Work out the finished part from the listing and answer in its coordinate system (mm). A direction names the side the tool comes from. Coordinates: 2 decimals unless noted, no trailing zeros. Loops run counter-clockwise (first coordinate to the right, second up) from the corner with the lowest first, then second, coordinate; pieces in that order, holes last. Notation, with made-up numbers: M 78,-13.5 L 136,-13.5 A24 ccw 136,20.5 Z; hole C 59.5,26.25 d8. An arc over 180 degrees is marked long. Write each question's results on one line, items separated by ' | '.
```python
from build123d import *

# Parameters (mm, degrees)
EXTRUDE1_DEPTH             = 75.692
SKETCH2_W                  = 7.9502
SKETCH2_H                  = 18.2626
SKETCH2_W_2                = 7.9248
EXTRUDE2_DEPTH             = 33.4772
EXTRUDE3_REACH             = 33.89
SKETCH3_W                  = 59.817
SKETCH3_H                  = 1.5875
EXTRUDE3_DIRECTION_2_REACH = 3.588
SKETCH4_W                  = 3.175
SKETCH4_H                  = 6.3373
EXTRUDE4_DEPTH             = 1.5875
SKETCH5_R                  = 4.0005
SKETCH5_R_2                = 1.1938
SKETCH5_R_3                = 2.1844
EXTRUDE5_DEPTH             = 1.5875
SKETCH6_R                  = 2.1844
SKETCH6_R_2                = 1.5875
EXTRUDE6_DEPTH             = 43.8498
FILLET1_R                  = 2.54
FILLET2_R                  = 0.254
FILLET3_R                  = 2.54
FILLET4_R                  = 2.54


with BuildPart() as part:
    # Sketch1 → Extrude1 (new body)
    with BuildSketch(Plane(origin=(0, 0, 0), x_dir=(0, 0, -1), z_dir=(1, 0, 0))):
        with BuildLine():
            Line((1.5875, 33.4772), (1.5875, 1.5875))
            Line((1.5875, 1.5875), (41.2623, 1.5875))
            Line((41.2623, 1.5875), (41.2623, 33.4772))
            Line((41.2623, 33.4772), (42.8498, 33.4772))
            Line((42.8498, 33.4772), (42.8498, 1.5875))
            ThreePointArc((42.8498, 1.5875), (42.384832015, 0.464967985), (41.2623, 0))
            Line((41.2623, 0), (1.5875, 0))
            ThreePointArc((1.5875, 0), (0.464967985, 0.464967985), (0, 1.5875))
            Line((0, 1.5875), (0, 33.4772))
            Line((0, 33.4772), (1.5875, 33.4772))
        make_face()
    extrude(amount=EXTRUDE1_DEPTH)

    # Sketch2 → Extrude2 (cut)
    with BuildSketch(Plane(origin=(0, 33.4772, 0), x_dir=(1, 0, 0), z_dir=(0, 1, 0))):
        with Locations((3.9751, 9.1313)):
            Rectangle(SKETCH2_W, SKETCH2_H)
        with Locations((71.7296, 9.1313)):
            Rectangle(SKETCH2_W_2, SKETCH2_H)
    extrude(amount=-EXTRUDE2_DEPTH, mode=Mode.SUBTRACT)

    # Extrude3: up to this face of the body (flat: up to its plane)
    extrude3_end = Plane(part.part.faces().sort_by_distance((37.846, 33.4772, -42.05605))[0])
    # Sketch3 → Extrude3 (cut, up to the picked face)
    with BuildSketch(Plane(origin=(0, 1.5875, 0), x_dir=(1, 0, 0), z_dir=(0, 1, 0)), mode=Mode.PRIVATE) as extrude3_sk1:
        with Locations((37.8587, 42.05605)):
            Rectangle(SKETCH3_W, SKETCH3_H)
    extrude3_tool1 = split(extrude(extrude3_sk1.sketch, amount=EXTRUDE3_REACH, mode=Mode.PRIVATE), bisect_by=extrude3_end, keep=Keep.BOTH, mode=Mode.PRIVATE)
    add(extrude3_tool1.solids().sort_by(Axis((37.8587, 1.5875, -42.05605), (0, 1, 0)))[0], mode=Mode.SUBTRACT)

    # Extrude3 direction 2: up to this face of the body (flat: up to its plane)
    extrude3_direction_2_end = Plane(part.part.faces().sort_by_distance((37.850626027, 0, -22.536595268))[0])
    # Sketch3 → Extrude3 direction 2 (cut, up to the picked face)
    with BuildSketch(Plane(origin=(0, 1.5875, 0), x_dir=(1, 0, 0), z_dir=(0, 1, 0)), mode=Mode.PRIVATE) as extrude3_direction_2_sk1:
        with Locations((37.8587, 42.05605)):
            Rectangle(SKETCH3_W, SKETCH3_H)
    extrude3_direction_2_tool1 = split(extrude(extrude3_direction_2_sk1.sketch, amount=-EXTRUDE3_DIRECTION_2_REACH, mode=Mode.PRIVATE), bisect_by=extrude3_direction_2_end, keep=Keep.BOTH, mode=Mode.PRIVATE)
    add(extrude3_direction_2_tool1.solids().sort_by(Axis((37.8587, 1.5875, -42.05605), (0, -1, 0)))[0], mode=Mode.SUBTRACT)

    # Sketch4 → Extrude4 (cut)
    with BuildSketch(Plane(origin=(0, 1.5875, 0), x_dir=(1, 0, 0), z_dir=(0, 1, 0))):
        with Locations((9.5377, 38.09365)):
            Rectangle(SKETCH4_W, SKETCH4_H)
        with Locations((66.1797, 38.09365)):
            Rectangle(SKETCH4_W, SKETCH4_H)
    extrude(amount=-EXTRUDE4_DEPTH, mode=Mode.SUBTRACT)

    # Sketch5 → Extrude5 (cut)
    with BuildSketch(Plane(origin=(0, 1.5875, 0), x_dir=(1, 0, 0), z_dir=(0, 1, 0))):
        with Locations(Location((21.1836, 29.1592, 0), (0, 0, 270))):  # turned: the seam where the file's is
            Circle(SKETCH5_R)
        with Locations(Location((21.1836, 37.4904, 0), (0, 0, 270))):  # turned: the seam where the file's is
            Circle(SKETCH5_R_2)
        with Locations(Location((12.8524, 29.1592, 0), (0, 0, 270))):  # turned: the seam where the file's is
            Circle(SKETCH5_R_2)
        with Locations(Location((21.1836, 20.828, 0), (0, 0, 270))):  # turned: the seam where the file's is
            Circle(SKETCH5_R_2)
        with Locations(Location((37.846, 37.4904, 0), (0, 0, 270))):  # turned: the seam where the file's is
            Circle(SKETCH5_R_2)
        with Locations(Location((29.5148, 29.1592, 0), (0, 0, 270))):  # turned: the seam where the file's is
            Circle(SKETCH5_R_2)
        with Locations(Location((37.846, 20.828, 0), (0, 0, 270))):  # turned: the seam where the file's is
            Circle(SKETCH5_R_2)
        with Locations(Location((37.846, 29.1592, 0), (0, 0, 270))):  # turned: the seam where the file's is
            Circle(SKETCH5_R)
        with Locations(Location((54.5084, 20.828, 0), (0, 0, 270))):  # turned: the seam where the file's is
            Circle(SKETCH5_R_2)
        with Locations(Location((54.5084, 29.1592, 0), (0, 0, 270))):  # turned: the seam where the file's is
            Circle(SKETCH5_R)
        with Locations(Location((46.1772, 29.1592, 0), (0, 0, 270))):  # turned: the seam where the file's is
            Circle(SKETCH5_R_2)
        with Locations(Location((54.5084, 37.4904, 0), (0, 0, 270))):  # turned: the seam where the file's is
            Circle(SKETCH5_R_2)
        with Locations(Location((62.8396, 29.1592, 0), (0, 0, 270))):  # turned: the seam where the file's is
            Circle(SKETCH5_R_2)
        with Locations(Location((3.7592, 29.1592, 0), (0, 0, 270))):  # turned: the seam where the file's is
            Circle(SKETCH5_R_3)
        with Locations(Location((71.9328, 29.1592, 0), (0, 0, 270))):  # turned: the seam where the file's is
            Circle(SKETCH5_R_3)
    extrude(amount=-EXTRUDE5_DEPTH, mode=Mode.SUBTRACT)

    # Sketch6 → Extrude6 (cut, through all)
    with BuildSketch(Plane.XY):
        with Locations((3.7592, 27.0002)):
            Circle(SKETCH6_R)
        with Locations((3.7592, 11.1252)):
            Circle(SKETCH6_R)
        with Locations((71.9328, 27.0002)):
            Circle(SKETCH6_R)
        with Locations((71.9328, 11.1252)):
            Circle(SKETCH6_R)
        with Locations((22.0726, 19.05)):
            Circle(SKETCH6_R_2)
        with Locations((53.6194, 19.05)):
            Circle(SKETCH6_R_2)
    extrude(amount=-EXTRUDE6_DEPTH, mode=Mode.SUBTRACT)

    # Fillet1
    fillet1_edges = [part.edges().sort_by_distance(p)[0] for p in [
        (64.5922, 0.79375, -41.2623),
        (0, 33.4772, -42.05605),
        (7.9502, 33.4772, -0.79375),
        (75.692, 33.4772, -42.05605),
        (75.692, 0.79375, -18.2626),
        (67.7672, 33.4772, -0.79375),
        (11.1252, 0.79375, -41.2623),
    ]]
    fillet(fillet1_edges, radius=FILLET1_R)

    # Fillet2
    fillet2_edges = [part.edges().sort_by_distance(p)[0] for p in [
        (71.7296, 1.5875, -41.2623),
        (37.8587, 1.5875, -1.5875),
        (3.9751, 1.5875, -41.2623),
    ]]
    fillet(fillet2_edges, radius=FILLET2_R)

    # Fillet3
    fillet3_edges = [part.edges().sort_by_distance(p)[0] for p in [
        (0, 0.79375, -18.2626),
    ]]
    fillet(fillet3_edges, radius=FILLET3_R)

    # Fillet4
    fillet4_edges = [part.edges().sort_by_distance(p)[0] for p in [
        (67.7672, 33.4772, -42.05605),
        (7.9502, 33.4772, -42.05605),
    ]]
    fillet(fillet4_edges, radius=FILLET4_R)


solid = part.part
```
1) Find section D-D, the plane z = -23. Give the vertices of the cut face in (x, y), and give its area (3 significant figures).
Check result:
outline: M 0,0 L 75.69,0 L 75.69,1.59 L 0,1.59 Z | area: 120 mm^2
2) Straight lines are drawn through the part: probe 1 along Z at (x, y) = (55, 8.5); probe 2 along Y at (x, z) = (28, -3). For each, find the intervals that lie inside material, in ascending order. Write a range as [from, to].
Check result:
probe 1: [-1.59, 0] | probe 2: [0, 1.59]
3) For a pull along X with two mould halves and no side action, classify faces 4 (the face through (0.72, 32.71, -42.07)), 5 (the face through (37.44, 0.45, -0.48)), 6 (the face through (30.32, 0.8, -30.04)) as released by +X, released by -X, zero draft, split by the parting line, or undercut.
Check result:
face 4: released by -X | face 5: zero draft | face 6: undercut
4) Find section C-C, the plane z = -16.5. Give the vertices of the cut face in (x, y), and give its area (3 significant figures).
Check result:
outline: M 7.95,0 L 67.77,0 L 67.77,1.59 L 7.95,1.59 Z | area: 95.0 mm^2
5) Find section A-A, the plane y = 22. Give the vertices of the cut face in (x, z).
Check result:
outline: M 0,-42.85 L 7.95,-42.85 L 7.95,-41.26 L 0,-41.26 Z; M 7.95,-1.59 L 67.77,-1.59 L 67.77,0 L 7.95,0 Z; M 67.77,-42.85 L 75.69,-42.85 L 75.69,-41.26 L 67.77,-41.26 Z
6) Given pin 1 Ø4 at (x, y) = (73, 18.5) entering from +Z; pin 2 Ø0.8 at (x, y) = (10, 1) entering from -Z (3 decimals); pin 3 Ø4 at (x, z) = (49.5, -20) entering from +Y, each flat-ended and moving along its own axis, determine where each tip first touches the part or whether it passes through.
Check result:
pin 1: z = -41.26 | pin 2: z = -34.925 | pin 3: y = 1.59
7) Which of the six approach directions +Z, -Z, +X, -X, +Y, -Y give full straight-line access (tool end or side, diameter ignored) to faces 1 (the face through (70, 1, -18.263)), 2 (the face through (4, 17, -41.262)), 3 (the face through (7.95, 13, -42))?
Check result:
face 1: +Z, +X, +Y, -Y | face 2: +Z, +X, -X, +Y | face 3: -Z, +Y, -Y
